Design review of the part built by this model. Coordinates are the model's own, in mm. A direction names the side the tool comes from. Give positions to 0.01 mm unless a question says otherwise; leave off trailing zeros. Write each loop counter-clockwise with the first axis right and the second up, starting at its lowest first coordinate (ties: lowest second). Pieces come first, ordered by that corner, then holes. Notation, with made-up numbers: (69, 48.25) -> (93, 48.25) arc R25 ccw to (93, 60.25) -> close; hole circle Ø2 at (15, 15). An arc over 180 degrees is marked (long way). Use CSV: the item, a comma, the result in double quotes.
Autodesk Inventor part; units mm, degrees
ref_plane "YZ Plane" through (0, 0, 0) normal (1, 0, 0) x (0, 1, 0)
ref_plane "XZ Plane" through (0, 0, 0) normal (0, 1, 0) x (-1, 0, 0)
ref_plane "XY Plane" through (0, 0, 0) normal (0, 0, 1) x (1, 0, 0)
sketch "Эскиз1" plane through (0, 0, 0) normal (0, 1, 0) x (-1, 0, 0)
  line L0 (19.5, 0) -> (12.5, 0)
  line L1 (12.5, 0) -> (12.5, -40.5)
  line L2 (12.5, -40.5) -> (19.5, -40.5)
  line L3 (19.5, -40.5) -> (19.5, 0)
  line L4 (-12.5, 0) -> (-19.5, 0)
  line L5 (-19.5, 0) -> (-19.5, -40.5)
  line L6 (-19.5, -40.5) -> (-12.5, -40.5)
  line L7 (-12.5, -40.5) -> (-12.5, 0)
  line L8 (0, 0) -> (0, -102.7933) construction
  line L9 (12.5, -7) -> (15.5, -7)
  line L10 (15.5, -7) -> (15.5, -9.5)
  line L11 (15.5, -9.5) -> (12.5, -9.5)
  line L12 (12.5, -9.5) -> (12.5, -7)
  line L13 (-12.5, -7) -> (-15.5, -7)
  line L14 (-15.5, -7) -> (-15.5, -9.5)
  line L15 (-15.5, -9.5) -> (-12.5, -9.5)
  line L16 (-12.5, -9.5) -> (-12.5, -7)
  line L17 (15.5, -21.5) -> (12.5, -21.5)
  line L18 (12.5, -19) -> (15.5, -19)
  line L19 (15.5, -19) -> (15.5, -21.5)
  line L20 (12.5, -21.5) -> (12.5, -19)
  line L21 (-15.5, -21.5) -> (-12.5, -21.5)
  line L22 (-15.5, -19) -> (-15.5, -21.5)
  line L23 (-12.5, -19) -> (-15.5, -19)
  line L24 (-12.5, -21.5) -> (-12.5, -19)
  line L25 (15.5, -33.5) -> (12.5, -33.5)
  line L26 (12.5, -31) -> (15.5, -31)
  line L27 (15.5, -31) -> (15.5, -33.5)
  line L28 (12.5, -33.5) -> (12.5, -31)
  line L29 (-15.5, -33.5) -> (-12.5, -33.5)
  line L30 (-15.5, -31) -> (-15.5, -33.5)
  line L31 (-12.5, -31) -> (-15.5, -31)
  line L32 (-12.5, -33.5) -> (-12.5, -31)
  line L33 (19.5, 0) -> (-19.5, 0)
  line L34 (-12.5, -5) -> (12.5, -5)
  line L35 (-19.5, -40.5) -> (19.5, -40.5)
  line L36 (12.5, -35.5) -> (-12.5, -35.5)
  line L37 (12.5, -11.5) -> (-12.5, -11.5)
  line L38 (-12.5, -11.5) -> (-12.5, -17)
  line L39 (-12.5, -17) -> (12.5, -17)
  line L40 (12.5, -17) -> (12.5, -11.5)
  line L41 (12.5, -23.5) -> (-12.5, -23.5)
  line L42 (-12.5, -23.5) -> (-12.5, -29)
  line L43 (-12.5, -29) -> (12.5, -29)
  line L44 (12.5, -29) -> (12.5, -23.5)
  line L45 (19.5, -11.5) -> (17.5, -11.5)
  line L46 (17.5, -11.5) -> (17.5, -17)
  line L47 (17.5, -17) -> (19.5, -17)
  line L48 (19.5, -17) -> (19.5, -11.5)
  line L49 (19.5, -23.5) -> (17.5, -23.5)
  line L50 (17.5, -23.5) -> (17.5, -29)
  line L51 (17.5, -29) -> (19.5, -29)
  line L52 (19.5, -29) -> (19.5, -23.5)
  line L53 (-19.5, -11.5) -> (-17.5, -11.5)
  line L54 (-17.5, -11.5) -> (-17.5, -17)
  line L55 (-17.5, -17) -> (-19.5, -17)
  line L56 (-19.5, -17) -> (-19.5, -11.5)
  line L57 (-19.5, -23.5) -> (-17.5, -23.5)
  line L58 (-17.5, -23.5) -> (-17.5, -29)
  line L59 (-17.5, -29) -> (-19.5, -29)
  line L60 (-19.5, -29) -> (-19.5, -23.5)
  line L61 (2.75, 0) -> (-2.75, 0)
  line L62 (-2.75, 0) -> (-2.75, -2)
  line L63 (-2.75, -2) -> (2.75, -2)
  line L64 (2.75, -2) -> (2.75, 0)
  line L65 (2.75, -40.5) -> (-2.75, -40.5)
  line L66 (-2.75, -40.5) -> (-2.75, -38.5)
  line L67 (-2.75, -38.5) -> (2.75, -38.5)
  line L68 (2.75, -38.5) -> (2.75, -40.5)
  point P0 (-12.5, -40.5)
  point P1 (-12.5, -33.5)
  point P2 (-12.5, -31)
  point P3 (-12.5, -21.5)
  point P4 (-12.5, -19)
  point P5 (-12.5, -9.5)
  point P6 (12.5, -9.5)
  point P7 (12.5, -19)
  point P8 (12.5, -21.5)
  point P9 (12.5, -31)
  point P10 (12.5, -33.5)
  point P11 (12.5, -29)
  point P12 (12.5, -17)
  point P13 (-12.5, -11.5)
  point P14 (18.5, -17)
  point P15 (18.5, -11.5)
  point P16 (-18.5, -11.5)
  point P17 (-18.5, -17)
  point P18 (-18.5, -23.5)
  point P19 (18.5, -23.5)
  point P20 (-19.5, -17)
  point P21 (-19.5, -29)
  point P22 (19.5, -17)
  dimension "d0" = 2.5
  dimension "d1" = 3
  dimension "d4" = 12
  dimension "d9" = 31
  dimension "d10" = 4
  dimension "d11" = 5
  dimension "d12" = 5
  dimension "d14" = 2
  dimension "d17" = 2
  dimension "d18" = 2
  dimension "d19" = 2
  dimension "d20" = 2
  dimension "d21" = 2
  dimension "d24" = 2
  dimension "d25" = 2
  dimension "d26" = 5.5
extrude "Выдавливание1" add sketch "Эскиз1" along normal blind 3 contours L3 L45 L46 L47 L49 L50 L51 L2 L1 L25 L27 L26 L17 L19 L18 L11 L10 L9 L0 | L1 L34 L7 L33 L62 L63 L64 | L7 L13 L14 L15 L23 L22 L21 L31 L30 L29 L6 L5 L59 L58 L57 L55 L54 L53 L4 | L1 L39 L7 L37 | L35 L68 L67 L66 L7 L36 L1 | L1 L43 L7 L41
fillet "Сопряжение1" radius 2 12 edges at (12.5, 1.5, -5) (-12.5, 1.5, -5) (-12.5, 1.5, -11.5) (12.5, 1.5, -11.5) (12.5, 1.5, -23.5) (12.5, 1.5, -35.5) (12.5, 1.5, -17) (12.5, 1.5, -29) (-12.5, 1.5, -17) (-12.5, 1.5, -23.5) (-12.5, 1.5, -35.5) (-12.5, 1.5, -29)
fillet "Сопряжение2" radius 5 4 edges at (-19.5, 1.5, 0) (19.5, 1.5, 0) (19.5, 1.5, -40.5) (-19.5, 1.5, -40.5)
equation "\"d12\" = d11"
properties part number "Крепление РБАСУ" material "Пластик АБС"
(1) Mouldability with a two-part tool opening along Z and no side actions: class faces 1 (the face through (18.07, 1.52, -39)), 2 (the face through (14, 1, -21.5)), 3 (the face through (-2.75, 1, -39)) as +Z half, -Z half, draft (parallel to the pull), parting line (faces both ways), or undercut.
Established:
face 1,"-Z half"
face 2,"undercut"
face 3,"draft"
(2) For line 1 along Z through (x, y) = (-13, 0.2); line 2 along Z through (x, y) = (-3.5, 0.9); line 3 along X through (y, z) = (1.6, -31.5), list the stretches that pass through material, from the lowest coordinate up. Write a range as [from, to].
Established:
line 1,"z = [-40.5, -33.5], [-31, -21.5], [-19, -9.5], [-7, 0]"
line 2,"z = [-40.5, -35.5], [-29, -23.5], [-17, -11.5], [-5, 0]"
line 3,"x = [-19.5, -15.5], [15.5, 19.5]"
(3) Take a section at B-B (z = -23). Write out the cut boundary in (x, y).
Established:
outline,"(-19.5, 0) -> (-11.82, 0) -> (-11.82, 3) -> (-19.5, 3) -> close; (11.82, 0) -> (19.5, 0) -> (19.5, 3) -> (11.82, 3) -> close"
(4) Clearance check with flat-ended pins moving along their axes: pin 1 (0.9 mm diameter, centred on y = 2, z = -25.5, fed in from -X); pin 2 (0.6 mm diameter, centred on y = 1.5, z = -1, fed in from -X); pin 3 (0.6 mm diameter, centred on x = 18, y = 1, fed in from +Z). State where each tip first meets the part, or that it passes through.
Established:
pin 1,"stops at x = -17.5"
pin 2,"stops at x = -17.86"
pin 3,"stops at z = -1.16"
(5) Take a section at A-A (x = 13). Write out the cut boundary in (y, z), then the cut area to 3 significant figures.
Established:
outline,"(0, -40.5) -> (3, -40.5) -> (3, -33.5) -> (0, -33.5) -> close; (0, -31) -> (3, -31) -> (3, -21.5) -> (0, -21.5) -> close; (0, -19) -> (3, -19) -> (3, -9.5) -> (0, -9.5) -> close; (0, -7) -> (3, -7) -> (3, 0) -> (0, 0) -> close"
area,"99.0 mm2"
(6) Take a section at C-C (x = 0.5). Write out the cut boundary in (y, z), then the cut area to 3 significant figures.
Established:
outline,"(0, -38.5) -> (3, -38.5) -> (3, -35.5) -> (0, -35.5) -> close; (0, -29) -> (3, -29) -> (3, -23.5) -> (0, -23.5) -> close; (0, -17) -> (3, -17) -> (3, -11.5) -> (0, -11.5) -> close; (0, -5) -> (3, -5) -> (3, -2) -> (0, -2) -> close"
area,"51.0 mm2"
(7) Tool access review of faces 4 (the face through (19, 1, -11.5)), 5 (the face through (-17.5, 1, -26)), 6 (the face through (-14, 1, -31)): name each direction out of +Z, -Z, +X, -X, +Y, -Y from which nothing blocks a thin tool from reaching the whole face with its end or side.
Established:
face 4,"+X, +Y, -Y"
face 5,"-X, +Y, -Y"
face 6,"+Y, -Y"
(8) Take a section at D-D (y = 1.5). State how many separate pieces and enclosed holes the cut face has, then the cut area to 3 significant figures.
Established:
separate pieces,"1"
enclosed holes,"3"
area,"970 mm2"
